Could you check a few things on this model? Use its own coordinates, in mm. A direction names the side the tool comes from. Give positions to 0.01 mm unless a question says otherwise; leave off trailing zeros. Order: outer loops, then holes, each group sorted by start corner. A loop starts at its lowest first (then second) coordinate and runs counter-clockwise, first axis right, second up. Notation, with made-up numbers: (79.5, 83.25) - (100.5, 83.25) arc R25 ccw to (100.5, 107.25) - close; hole circle Ø11 at (-39, 24). An arc over 180 degrees is marked (long way). Put each result on its own line as item: value.
from build123d import *

# Parameters (mm, degrees)
F0_R     = 12.5
F1_DEPTH = 175
F2_R     = 20
F3_DEPTH = 10
F4_R     = 12.5
F5_DEPTH = 10
F6_R     = 2.5
F7_R     = 2.5
F8_DEPTH = 12.5
F9_R     = 1
F10_R    = 5


with BuildPart() as f1:
    # F0 (on Right) → F1 (new body)
    with BuildSketch(Plane.YZ):
        Circle(F0_R)
    extrude(amount=F1_DEPTH)

    # F2 (on face) → F3 (join)
    with BuildSketch(Plane.YZ.offset(175)):
        Circle(F2_R)
    extrude(amount=F3_DEPTH)

    # F4 (on face) → F5 (join)
    with BuildSketch(Plane.YZ.offset(185)):
        Circle(F4_R)
    extrude(amount=F5_DEPTH)

    # F6
    f6_edges = [f1.edges().sort_by_distance(p)[0] for p in [
        (195, -12.5, 0),
        (185, -20, 0),
    ]]
    fillet(f6_edges, radius=F6_R)

    # F7 (on Front) → F8 (cut, symmetric)
    with BuildSketch(Plane.XZ):
        with Locations((22.5, 0)):
            Circle(F7_R)
    extrude(amount=F8_DEPTH, both=True, mode=Mode.SUBTRACT)

    # F9
    f9_edges = [f1.edges().sort_by_distance(p)[0] for p in [
        (22.5, 12.247449, 2.5),
        (22.5, 12.247449, -2.5),
        (20, -12.5, 0),
    ]]
    fillet(f9_edges, radius=F9_R)

    # F10
    f10_edges = [f1.edges().sort_by_distance(p)[0] for p in [
        (0, -12.5, 0),
    ]]
    fillet(f10_edges, radius=F10_R)


solid = f1.part
1) Suppose I cut it at A-A, the plane y = 0. List the corners of the cut face in (x, z) for me, and give its area (3 significant figures).
Filled in:
outline: (0, -7.5) arc R5 ccw to (5, -12.5) - (175, -12.5) - (175, -20) - (182.5, -20) arc R2.5 ccw to (185, -17.5) - (185, -12.5) - (192.5, -12.5) arc R2.5 ccw to (195, -10) - (195, 10) arc R2.5 ccw to (192.5, 12.5) - (185, 12.5) - (185, 17.5) arc R2.5 ccw to (182.5, 20) - (175, 20) - (175, 12.5) - (5, 12.5) arc R5 ccw to (0, 7.5) - close; hole circle Ø5 at (22.5, 0)
area: 4,990 mm^2
2) We'd pull the mould along Z, two halves only. Please class faces 1 (the cylindrical face through (88.81, 11.923, 3.755)), 2 (the flat face through (195, 0, 0)), 3 (the cylindrical face through (20, 0, 0)): pulls with the +Z half, pulls with the -Z half, needs draft (parallel to the pull), parting line crosses it, or undercut.
Filled in:
face 1: parting line crosses it
face 2: needs draft
face 3: undercut
3) If I drill on line 1 (X direction, y = 5.25, z = 0); line 2 (Y direction, x = 55.5, z = 10); line 3 (Z direction, x = 22, y = -4), over which ranges is the centre line in solid material (lowest first)? Write a range as [from, to].
Filled in:
line 1: x = [0, 20], [25, 195]
line 2: y = [-7.5, 7.5]
line 3: z = [-11.84, -2.45], [2.45, 11.84]
4) Which directions (+Z, -Z, +X, -X, +Y, -Y) give clear straight access to the entire face, cutting with the end or side of a thin tool? Please do faces 4 (the cylindrical face through (188.698, 11.923, 3.755)), 5 (the flat face through (175, 9, 9)), 6 (the cylindrical face through (178.698, -4.336, -19.524)).
Filled in:
face 4: +X
face 5: -X
face 6: +X, -X
5) Suppose I cut it at B-B, the plane x = 127. List the corners of the cut face in (y, z) for me, and give its area (3 significant figures).
Filled in:
outline: circle Ø25 at (0, 0)
area: 491 mm^2
6) I'm going to push flat-ended pins straight in: pin 1 (8 mm diameter, centred on y = -11.5, z = -8.5, fed in from -X); pin 2 (4 mm diameter, centred on x = 40.5, y = 8.5, fed in from +Z); pin 3 (4 mm diameter, centred on y = 9, z = -4.5, fed in from -X). Where does each tip first touch, or does it pass through?
Filled in:
pin 1: stops at x = 0.86
pin 2: stops at z = 10.68
pin 3: stops at x = 0.03
